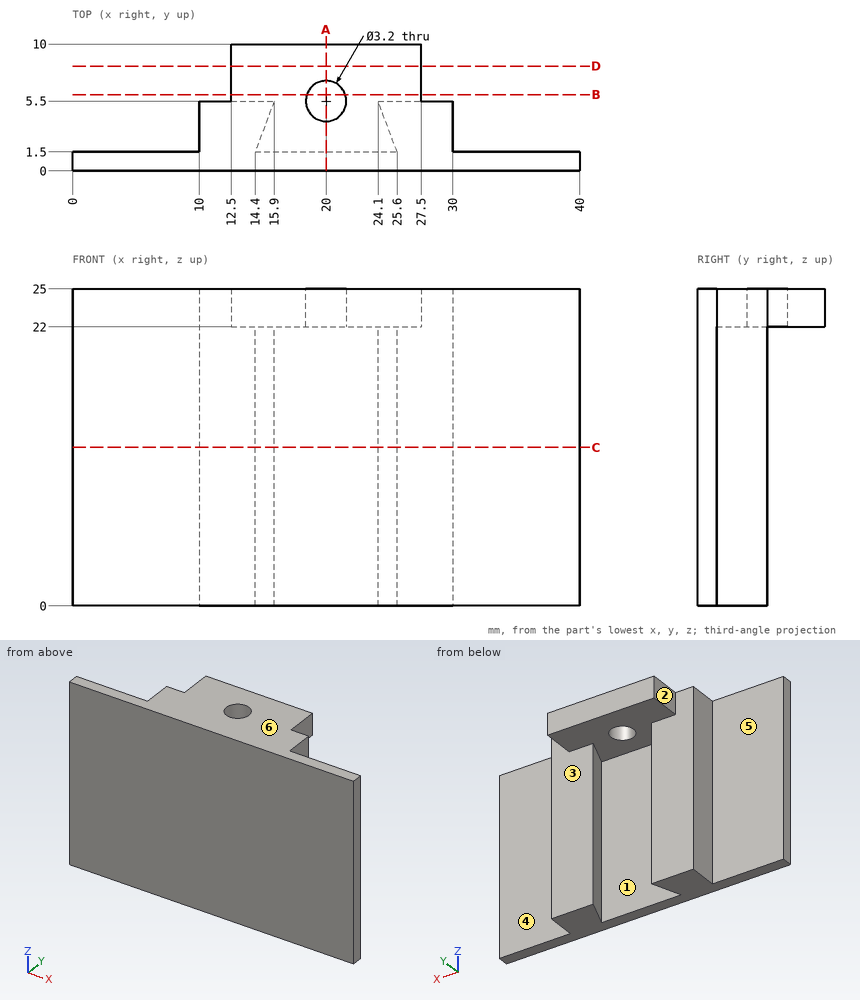
Can you work these out from the drawing? Everything is in mm from the part's minimum corner. A direction names the side the tool comes from. Round coordinates to 2 decimals unless told otherwise and drop trailing zeros. Loops run counter-clockwise (first coordinate to the right, second up) from the corner with the lowest first, then second, coordinate; pieces in that order, holes last. Notation, with made-up numbers: (79.5, 20.5) - (133.5, 20.5) arc R17 ccw to (133.5, 29.5) - close; hole circle Ø3 at (51.25, 16). An arc over 180 degrees is marked (long way). One line per question, with ' | ' between items. Start each with the question number.
Q1. We'd pull the mould along X, two halves only. Please class the marked faces 1, 2 and 3: +X half, -X half, draft (parallel to the pull), parting line (faces both ways), or undercut.
Q2. I want a section at C-C (z = 12.5). Write out the boundary of the cut face in (x, y), then the cut area to 3 significant figures.
Q3. I want a section at A-A (x = 20). Write out the boundary of the cut face in (y, z), then the cut area to 3 significant figures.
Q4. Please list where these lines run through material, in increasing order: line 1 (Y direction, x = 20, z = 24.35); line 2 (Z direction, x = 22.5, y = 9); line 3 (Y direction, x = 29, z = 11). Write a range as [from, to].
Q5. Will these pins go through, and if not, where does the flat tip stop? pin 1 (5 mm diameter, centred on x = 20, y = 5.5, fed in from -Z); pin 2 (3 mm diameter, centred on x = 16, z = 11.5, fed in from +Y); pin 3 (2 mm diameter, centred on y = 3, z = 20, fed in from +X).
Q6. I want a section at B-B (y = 6). Write out the boundary of the cut face in (x, z), then the cut area to 3 significant figures.
Q7. For the marked faces 4, 5 and 6, which set-ups out of +Z, -Z, +X, -X, +Y, -Y let a thin tool reach every point of the face, with its end or its side?
Q8. I want a section at D-D (y = 8.25). Write out the boundary of the cut face in (x, z).
Response values:
1) face 1: undercut | face 2: -X half | face 3: draft
2) outline: (0, 0) - (40, 0) - (40, 1.5) - (30, 1.5) - (30, 5.5) - (24.1, 5.5) - (25.6, 1.5) - (14.4, 1.5) - (15.9, 5.5) - (10, 5.5) - (10, 1.5) - (0, 1.5) - close | area: 101 mm²
3) outline: (0, 0) - (1.5, 0) - (1.5, 22) - (3.9, 22) - (3.9, 25) - (0, 25) - close; (7.1, 22) - (10, 22) - (10, 25) - (7.1, 25) - close | area: 53.4 mm²
4) line 1: y = [0, 3.9], [7.1, 10] | line 2: z = [22, 25] | line 3: y = [0, 5.5]
5) pin 1: stops at z = 22 | pin 2: stops at y = 5.5 | pin 3: stops at x = 30
6) outline: (12.5, 22) - (18.48, 22) - (18.48, 25) - (12.5, 25) - close; (21.52, 22) - (27.5, 22) - (27.5, 25) - (21.52, 25) - close | area: 35.9 mm²
7) face 4: +Z, -Z, +X, +Y | face 5: +Z, -Z, -X, +Y | face 6: +Z, +X, -X, +Y, -Y
8) outline: (12.5, 22) - (27.5, 22) - (27.5, 25) - (12.5, 25) - close
